```python
from build123d import *

# Parameters (mm, degrees)
ESTRUSIONE_ESTRUSIONE1_DEPTH = 819
SCHIZZO3_R                   = 1.7
TAGLIO_ESTRUSIONE1_DEPTH     = 821.494363174


with BuildPart() as part:
    # Schizzo2 → Estrusione-Estrusione1 (new body)
    with BuildSketch(Plane(origin=(0, 0, 0), x_dir=(1, 0, 0), z_dir=(0, 1, 0))):
        Polygon((0, 0), (35, 0), (35, 2), (2, 2), (2, 35), (0, 35), align=None)
    extrude(amount=ESTRUSIONE_ESTRUSIONE1_DEPTH)

    # Schizzo3 → Taglio-Estrusione1 (cut, through all)
    with BuildSketch(Plane.XY):
        with Locations((20, 20)):
            Circle(SCHIZZO3_R)
        with Locations((20, 330.4)):
            Circle(SCHIZZO3_R)
        with Locations((20, 485.6)):
            Circle(SCHIZZO3_R)
        with Locations((20, 175.2)):
            Circle(SCHIZZO3_R)
        with Locations((20, 640.8)):
            Circle(SCHIZZO3_R)
        with Locations((20, 799)):
            Circle(SCHIZZO3_R)
    extrude(amount=-TAGLIO_ESTRUSIONE1_DEPTH, mode=Mode.SUBTRACT)


solid = part.part
```
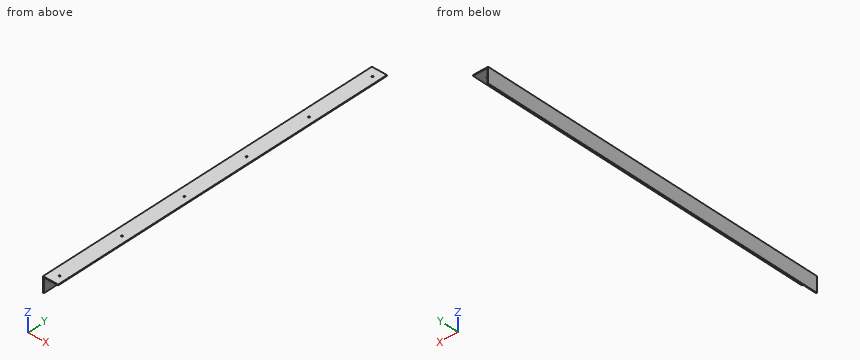
Model file for the job. Use its own axes, mm. Round coordinates to 2 decimals unless told otherwise and drop trailing zeros. Write each loop counter-clockwise with the first axis right and the second up, starting at its lowest first coordinate (ties: lowest second). Pieces come first, ordered by that corner, then holes. Notation, with made-up numbers: (12, 49.5) - (27, 49.5) arc R12 ccw to (27, 71.5) - close; hole circle Ø3 at (86.25, -19). An arc over 180 degrees is marked (long way). One line per item, written item: value.
(1) Cut at A-A, the plane z = -27.5. Give the cut face in (x, y).
Values follow:
outline: (0, 0) - (2, 0) - (2, 819) - (0, 819) - close
(2) Drop flat-ended pins along their axis: P1, Ø16.5, axis at y = 354.5, z = -14.5, coming from the +X side; P2, Ø4.5, axis at x = 20, y = 640.8, coming from the -Z side. Give the stop position or say it passes through.
Values follow:
P1: stops at x = 2
P2: stops at z = -2
(3) Cut at C-C, the plane x = 28. Give the cut face in (y, z), plus the area to 3 significant figures.
Values follow:
outline: (0, -2) - (819, -2) - (819, 0) - (0, 0) - close
area: 1,640 mm²
(4) Cut at B-B, the plane y = 440.5. Give the cut face in (x, z).
Values follow:
outline: (0, -35) - (2, -35) - (2, -2) - (35, -2) - (35, 0) - (0, 0) - close
(5) Wall check: probe 1 along X at (y, z) = (799, -0.9); probe 2 along Z at (x, y) = (9, 750); probe 3 along X at (y, z) = (599.5, -16.5). Give the ranges that are in metal, low to high.
Values follow:
probe 1: x = 0 to 18.3, 21.7 to 35
probe 2: z = -2 to 0
probe 3: x = 0 to 2
